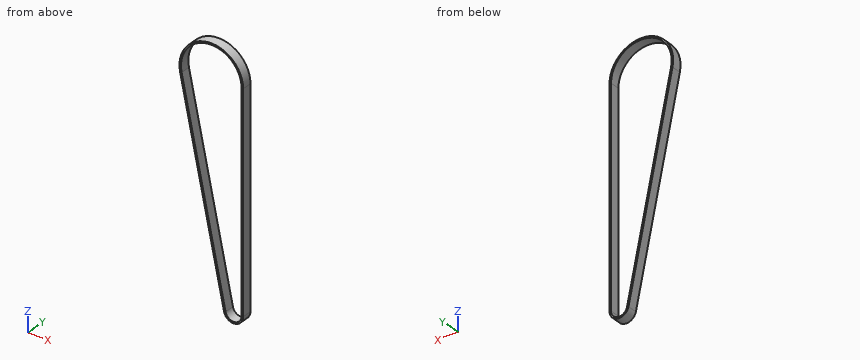
```python
from build123d import *

# Parameters (mm, degrees)
SKETCH_3_W = 1.5
SKETCH_3_H = 10


with BuildPart() as part:
    # 扫描1: sweep along a path in 草图2
    with BuildLine(Plane(origin=(0, 0, 0), x_dir=(1, 0, 0), z_dir=(0, 1, 0))) as sweep_1_path:
        Line((8, -212.5), (8, 0))
        ThreePointArc((8, 0), (0.823832006, 7.957468242), (-7.830325206, 1.638904257))
        Line((-7.830325206, 1.638904257), (-51.363719524, -206.354109038))
        ThreePointArc((-51.363719524, -206.354109038), (-25.089370023, -242.340505908), (8, -212.5))
    # 草图3 → 扫描1 (sweep)
    with BuildSketch(Plane.XY):
        with Locations((8.75, 5)):
            Rectangle(SKETCH_3_W, SKETCH_3_H)
    sweep(path=sweep_1_path.line)


solid = part.part
```
Read the model definition and answer for the solid it produces. Units are mm, in the model's axes. Coordinates: 2 decimals unless noted, no trailing zeros. Write each loop counter-clockwise with the first axis right and the second up, starting at its lowest first coordinate (ties: lowest second). Pieces come first, ordered by that corner, then holes. Notation, with made-up numbers: (41.25, -19) - (65.25, -19) arc R21 ccw to (65.25, -8) - close; hole circle Ø3 at (0.5, 49). An arc over 180 degrees is marked (long way). Answer as a JSON object with one key per item and string values. Group by question number.
1. A cutting plane is placed at C-C (z = 65.5). Determine the outline of the cut face in (x, y).
2. A cutting plane is placed at A-A (y = 3.25). Determine the outline of the cut face in (x, z), plus the area to 3 significant figures.
3. Each of these flat-tipped pins is pushed along its axis until it touches: P1, Ø6, axis at x = -38, y = 8, coming from the +Z side; P2, Ø1, axis at x = -30.5, y = 3, coming from the +Z side; P3, Ø5, axis at y = 3, z = 159, coming from the -X side; P4, Ø10, axis at x = -1, z = 133.5, coming from the +Y side. Where does it stop, or does it pass through?
4. Consider L1, parallel to X at y = 2, z = 26; L2, parallel to X at y = 2.75, z = 219. Determine where each line is inside the solid, lowest interval first. Write a range as [from, to].
5. A cutting plane is placed at B-B (x = -44). Determine the outline of the cut face in (y, z).
Worked out:
{
 "1": {"outline": "(-23.42, 0) - (-21.88, 0) - (-21.88, 10) - (-23.42, 10) - close; (8, 0) - (9.5, 0) - (9.5, 10) - (8, 10) - close"},
 "2": {"outline": "(-52.83, 206.05) - (-9.3, -1.95) arc R9.5 ccw to (9.5, 0) - (9.5, 212.5) arc R31.5 ccw (long way) to start; hole (-51.36, 206.35) - (-7.83, -1.64) arc R8 ccw to (8, 0) - (8, 212.5) arc R30 ccw (long way) to start", "area": "830 mm²"},
 "3": {"P1": "stops at z = 241.19", "P2": "stops at z = 242.97", "P3": "stops at x = -43.51", "P4": "passes through"},
 "4": {"L1": "x = [-15.15, -13.62], [8, 9.5]", "L2": "x = [-52.82, -51.29], [7.29, 8.82]"},
 "5": {"outline": "(0, 163.85) - (10, 163.85) - (10, 171.17) - (0, 171.17) - close; (0, 232.9) - (10, 232.9) - (10, 235.04) - (0, 235.04) - close"}
}
